from build123d import *

# Parameters (mm, degrees)
SKETCH1_R           = 6.5
BOSS_EXTRUDE1_DEPTH = 22
CAVITY1_START       = 2
CAVITY1_OUTLINE_R   = 5
CAVITY1_OUTLINE_R_2 = 0.75
CAVITY1_DEPTH       = 20
CAVITY1_START_2     = 17
CAVITY1_2_OUTLINE_R = 0.75
CAVITY1_2_DEPTH     = 5
SKETCH2_R           = 0.5
CUT_EXTRUDE1_DEPTH  = 23.011360703
SKETCH3_R           = 0.3
CUT_EXTRUDE2_DEPTH  = 23.011360703


# Read off the part's stored shape, not the designer's step: Cavity1
with BuildPart() as part:
    # Sketch1 → Boss-Extrude1 (new body)
    with BuildSketch(Plane(origin=(0, 0, 0), x_dir=(1, 0, 0), z_dir=(0, 1, 0))):
        with Locations(Location((0, 0, 0), (0, 0, 270))):
            Circle(SKETCH1_R)
    extrude(amount=BOSS_EXTRUDE1_DEPTH)

    # Cavity1 outline → Cavity1 (cut)
    with BuildSketch(Plane(origin=(0, 0, 0), x_dir=(1, 0, 0), z_dir=(0, 1, 0)).offset(CAVITY1_START)):
        Circle(CAVITY1_OUTLINE_R)
        Circle(CAVITY1_OUTLINE_R_2, mode=Mode.SUBTRACT)
        with BuildLine():
            ThreePointArc((2.598076211, 1.5), (0, 3), (-2.598076211, 1.5))
            Line((-2.598076211, 1.5), (-3.464101615, 2))
            ThreePointArc((-3.464101615, 2), (0, 4), (3.464101615, 2))
            Line((3.464101615, 2), (2.598076211, 1.5))
        make_face(mode=Mode.SUBTRACT)
    extrude(amount=CAVITY1_DEPTH, mode=Mode.SUBTRACT)

    # Cavity1 2 outline → Cavity1 2 (cut)
    with BuildSketch(Plane(origin=(0, 0, 0), x_dir=(1, 0, 0), z_dir=(0, 1, 0)).offset(CAVITY1_START_2)):
        Circle(CAVITY1_2_OUTLINE_R)
    extrude(amount=CAVITY1_2_DEPTH, mode=Mode.SUBTRACT)

    # Sketch2 → Cut-Extrude1 (cut, through all)
    with BuildSketch(Plane(origin=(0, 2, 0), x_dir=(1, 0, 0), z_dir=(0, 1, 0))):
        with Locations(Location((0, -3, 0), (0, 0, 270))):
            Circle(SKETCH2_R)
        with Locations(Location((-2.897777479, -0.776457135, 0), (0, 0, 270))):
            Circle(SKETCH2_R)
        with Locations(Location((2.897777479, -0.776457135, 0), (0, 0, 90))):
            Circle(SKETCH2_R)
    extrude(amount=-CUT_EXTRUDE1_DEPTH, mode=Mode.SUBTRACT)

    # Sketch3 → Cut-Extrude2 (cut, through all)
    with BuildSketch(Plane(origin=(0, 2, 0), x_dir=(1, 0, 0), z_dir=(0, 1, 0))):
        with Locations(Location((0, 4.5, 0), (0, 0, 270))):
            Circle(SKETCH3_R)
        with Locations(Location((3.181980515, 3.181980515, 0), (0, 0, 270))):
            Circle(SKETCH3_R)
        with Locations(Location((-3.181980515, 3.181980515, 0), (0, 0, 90))):
            Circle(SKETCH3_R)
    extrude(amount=-CUT_EXTRUDE2_DEPTH, mode=Mode.SUBTRACT)


solid = part.part
Design review of the part built by this model. Coordinates are the model's own, in mm. A direction names the side the tool comes from. Round coordinates to 2 decimals unless told otherwise and drop trailing zeros. Write each loop counter-clockwise with the first axis right and the second up, starting at its lowest first coordinate (ties: lowest second). Pieces come first, ordered by that corner, then holes.
Item 1: Wall thickness on L1, parallel to X at y = 15, z = 0; L2, parallel to Z at x = -3, y = 2.5; L3, parallel to Z at x = -2.5, y = 18.25: over which ranges is each line inside the solid? List them lowest first.
Item 2: Consider section A-A on y = 6.5. Give the boundary of the cut face in (x, z), and give its area (3 significant figures).
Item 3: Consider section D-D on z = -4.5. Give the boundary of the cut face in (x, y), and give its area (3 significant figures).
Item 4: Draft analysis for pull direction X (two halves, no side actions). For faces 3 (the flat face through (0, 17, 0)), 4 (the flat face through (0, 22, -3.3)), 5 (the cylindrical face through (-3.955, 10.846, -5.158)), state which applies: released by +X, released by -X, zero draft, split by the parting line, or undercut.
Item 5: Consider section B-B on x = 0. Give the boundary of the cut face in (y, z), and give its area (3 significant figures).
Item 6: For pin 1 Ø6 at (y, z) = (12.5, 2.5) entering from +X; pin 2 Ø3 at (y, z) = (3.5, 5) entering from +X; pin 3 Ø4 at (x, y) = (-3.5, 12.5) entering from -Z; pin 4 Ø2 at (x, y) = (3, 9.5) entering from -Z, all flat-tipped, find the tip position at first contact; note any pin that passes through.
Item 7: Consider section C-C on y = 17.5. Give the boundary of the cut face in (x, z).
Item 8: For faces 1 (the cylindrical face through (-0.75, 9.4, -0.03)), 2 (the cylindrical face through (-2.748, 1.014, 1.253)), list the 3-axis set-ups (+Z, -Z, +X, -X, +Y, -Y) from which the entire face can be reached by the end or side of a thin tool; tool diameter is ignored.
Check values:
1. L1: x = -6.5 to -5, -0.75 to 0.75, 5 to 6.5
1. L2: z = -5.77 to -4, -2.65 to -1.73, 4 to 5.77
1. L3: z = -6 to -4.33, -3.12 to -1.66, 4.33 to 6
2. outline: circle Ø13 at (0, 0); (-3.46, -2) arc R4 ccw to (3.46, -2) - (2.6, -1.5) arc R3 cw to (-2.6, -1.5) - close; circle Ø1.5 at (0, 0); hole circle Ø10 at (0, 0)
2. area: 63.3 mm2
3. outline: (-4.69, 0) - (-0.3, 0) - (-0.3, 2) - (-2.18, 2) - (-2.18, 22) - (-4.69, 22) - close; (0.3, 0) - (4.69, 0) - (4.69, 22) - (2.18, 22) - (2.18, 2) - (0.3, 2) - close
3. area: 118 mm2
4. face 3: undercut
4. face 4: zero draft
4. face 5: split by the parting line
5. outline: (0, -6.5) - (22, -6.5) - (22, -5) - (2, -5) - (2, -4.8) - (0, -4.8) - close; (0, -4.2) - (2, -4.2) - (2, -4) - (22, -4) - (22, -3) - (2, -3) - (2, -0.75) - (17, -0.75) - (17, 0.75) - (2, 0.75) - (2, 2.5) - (0, 2.5) - close; (0, 3.5) - (2, 3.5) - (2, 5) - (22, 5) - (22, 6.5) - (0, 6.5) - close
5. area: 125 mm2
6. pin 1: stops at x = 6.5
6. pin 2: stops at x = 5.48
6. pin 3: stops at z = -6.32
6. pin 4: stops at z = -6.18
7. outline: circle Ø13 at (0, 0); (-3.46, -2) arc R4 ccw to (3.46, -2) - (2.6, -1.5) arc R3 cw to (-2.6, -1.5) - close; hole circle Ø10 at (0, 0)
8. face 1: +Y
8. face 2: +Y, -Y
